```python
from build123d import *

# Parameters (mm, degrees)
SKETCH_W     = 30
SKETCH_H     = 12
PAD_DEPTH    = 1
SKETCH001_R  = 2.75
PAD001_DEPTH = 4
POCKET_DEPTH = 4


with BuildPart() as part:
    # Sketch → Pad (new body)
    with BuildSketch(Plane.XY):
        Rectangle(SKETCH_W, SKETCH_H)
    extrude(amount=PAD_DEPTH)

    # Sketch001 (on Face6 of Pad) → Pad001 (join)
    with BuildSketch(Plane.XY.offset(1)):
        Circle(SKETCH001_R)
        with Locations((-12, 0)):
            Circle(SKETCH001_R)
        with Locations((12, 0)):
            Circle(SKETCH001_R)
    extrude(amount=PAD001_DEPTH)

    # Sketch002 (on Face11 of Pad001) → Pocket (cut)
    with BuildSketch(Plane.XY.offset(5)):
        Polygon((-0.65, 2.05), (-0.65, 0.7), (-2.05, 0.7), (-2.05, -0.7), (-0.65, -0.7), (-0.65, -2.05), (0.65, -2.05), (0.65, -0.7), (2.05, -0.7), (2.05, 0.7), (0.65, 0.7), (0.65, 2.05), align=None)
        Polygon((-12.65, 2.05), (-12.65, 0.7), (-14.05, 0.7), (-14.05, -0.7), (-12.65, -0.7), (-12.65, -2.05), (-11.35, -2.05), (-11.35, -0.7), (-9.95, -0.7), (-9.95, 0.7), (-11.35, 0.7), (-11.35, 2.05), align=None)
    extrude(amount=-POCKET_DEPTH, mode=Mode.SUBTRACT)


solid = part.part
```
Can you work these out from the model? Positions are in its coordinate system, mm. A direction names the side the tool comes from. Round coordinates to 2 decimals unless told otherwise and drop trailing zeros. Loops run counter-clockwise (first coordinate to the right, second up) from the corner with the lowest first, then second, coordinate; pieces in that order, holes last. Notation, with made-up numbers: (40.25, 24) -> (72.25, 24) arc R37 ccw to (72.25, 63) -> close; hole circle Ø2 at (60, -39). An arc over 180 degrees is marked (long way). One line per item, written item: value. Start each with the question number.
1. If we mould it in two halves opening along Y, with no side actions, what happens to faces 3 (the cylindrical face through (-0.596, -2.685, 2.972)), 4 (the flat face through (-11, -1, 5)), 5 (the flat face through (-12.65, -1, 3)), 6 (the flat face through (-0.2, 6, 0.5))? For each: pulls with the +Y half, pulls with the -Y half, needs draft (parallel to the pull), parting line crosses it, or undercut.
2. If we section it at D-D, the plane y = 4.5: Write out the boundary of the cut face in (x, z), then the cut area to 3 significant figures.
3. For faces 1 (the flat face through (-0.2, -6, 0.5)), 2 (the flat face through (0.65, 1, 3)), which set-ups out of +Z, -Z, +X, -X, +Y, -Y let a thin tool reach every point of the face, with its end or its side?
4. For pin 1 (1.5 mm diameter, centred on y = -1, z = 3.5, fed in from -X); pin 2 (4.5 mm diameter, centred on x = -0.5, y = 0.5, fed in from +Z); pin 3 (1.1 mm diameter, centred on x = -13.5, z = 2.5, fed in from -Y); pin 4 (1 mm diameter, centred on x = -12, z = 2.5, fed in from -Y), each with a flat end and sliding along its axis, tell me the tip position at first contact or that it passes through.
5. If we section it at B-B, the plane y = 0: Write out the boundary of the cut face in (x, z), then the cut area to 3 significant figures.
6. If we section it at C-C, the plane x = 0: Write out the boundary of the cut face in (y, z), then the cut area to 3 significant figures.
7. If I drill on probe 1 along X at (y, z) = (0.75, 3.8); probe 2 along Z at (x, y) = (-10.5, 5); probe 3 along X at (y, z) = (-1.75, 3.25), over which ranges is the centre line in solid material (lowest first)?
8. If we section it at A-A, the plane z = 2: Write out the boundary of the cut face in (x, y).
Calculated:
1. face 3: parting line crosses it
1. face 4: needs draft
1. face 5: undercut
1. face 6: pulls with the +Y half
2. outline: (-15, 0) -> (15, 0) -> (15, 1) -> (-15, 1) -> close
2. area: 30.0 mm²
3. face 1: +Z, -Z, +X, -X, -Y
3. face 2: +Z
4. pin 1: stops at x = -14.74
4. pin 2: stops at z = 5
4. pin 3: stops at y = -2.58
4. pin 4: stops at y = -2.75
5. outline: (-15, 0) -> (15, 0) -> (15, 1) -> (14.75, 1) -> (14.75, 5) -> (9.25, 5) -> (9.25, 1) -> (2.75, 1) -> (2.75, 5) -> (2.05, 5) -> (2.05, 1) -> (-2.05, 1) -> (-2.05, 5) -> (-2.75, 5) -> (-2.75, 1) -> (-9.25, 1) -> (-9.25, 5) -> (-9.95, 5) -> (-9.95, 1) -> (-14.05, 1) -> (-14.05, 5) -> (-14.75, 5) -> (-14.75, 1) -> (-15, 1) -> close
5. area: 63.2 mm²
6. outline: (-6, 0) -> (6, 0) -> (6, 1) -> (2.75, 1) -> (2.75, 5) -> (2.05, 5) -> (2.05, 1) -> (-2.05, 1) -> (-2.05, 5) -> (-2.75, 5) -> (-2.75, 1) -> (-6, 1) -> close
6. area: 17.6 mm²
7. probe 1: x = -14.65 to -12.65, -11.35 to -9.35, -2.65 to -0.65, 0.65 to 2.65, 9.35 to 14.65
7. probe 2: z = 0 to 1
7. probe 3: x = -14.12 to -12.65, -11.35 to -9.88, -2.12 to -0.65, 0.65 to 2.12, 9.88 to 14.12
8. outline: circle Ø5.5 at (-12, 0); circle Ø5.5 at (0, 0); circle Ø5.5 at (12, 0); hole (-14.05, -0.7) -> (-12.65, -0.7) -> (-12.65, -2.05) -> (-11.35, -2.05) -> (-11.35, -0.7) -> (-9.95, -0.7) -> (-9.95, 0.7) -> (-11.35, 0.7) -> (-11.35, 2.05) -> (-12.65, 2.05) -> (-12.65, 0.7) -> (-14.05, 0.7) -> close; hole (-2.05, -0.7) -> (-0.65, -0.7) -> (-0.65, -2.05) -> (0.65, -2.05) -> (0.65, -0.7) -> (2.05, -0.7) -> (2.05, 0.7) -> (0.65, 0.7) -> (0.65, 2.05) -> (-0.65, 2.05) -> (-0.65, 0.7) -> (-2.05, 0.7) -> close
